Check sheet for the modelled part. Datum: model origin and axes. Units: mm. Face numbers are marked on the shaded views. Round coordinates to 2 decimals unless told otherwise and drop trailing zeros. Write each loop counter-clockwise with the first axis right and the second up, starting at its lowest first coordinate (ties: lowest second). Pieces come first, ordered by that corner, then holes.
Item 1: Go/stop test with flat-tipped pins: pin 1 Ø3 at (x, y) = (-20.22, 50.58) entering from +Z; pin 2 Ø6 at (y, z) = (54, -2) entering from +X; pin 3 Ø17.5 at (x, y) = (10, 58) entering from +Z; pin 4 Ø1 at (y, z) = (59, -2) entering from +X. Record where each tip stops, or that it passes through.
Item 2: Cross-section at D-D on z = -4. Enter the section's corners in (x, y).
Item 3: Cross-section at C-C on y = 64.58. Enter the section's corners in (x, z), plus the area to 3 significant figures.
Item 4: Release check for a two-part mould opening along X. For the marked faces 1, 2 and 3 record: +X half, -X half, draft (parallel to the pull), parting line (faces both ways), or undercut.
Item 5: Material ranges on line 1 (X direction, y = 58.5, z = -2.5); line 2 (X direction, y = 56, z = 3.75); line 3 (X direction, y = 56, z = -3), recorded low to high.
Item 6: Cross-section at B-B on z = 4.25. Enter the section's corners in (x, y).
Item 7: Cross-section at A-A on x = -20.22. Enter the section's corners in (y, z), plus the area to 3 significant figures.
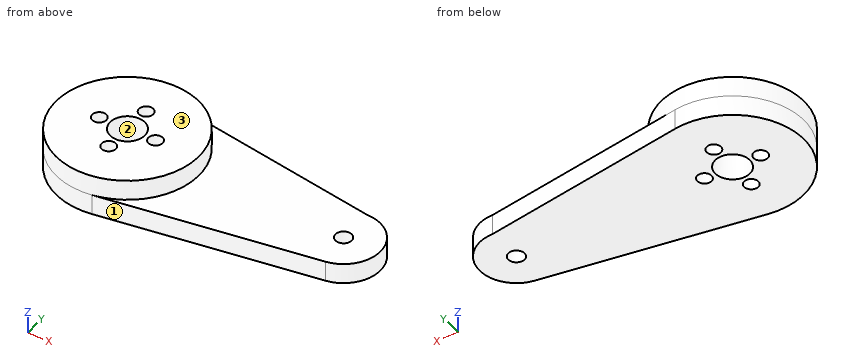
from build123d import *

# Parameters (mm, degrees)
SKETCH2_R           = 4.25
SKETCH2_R_2         = 2
BOSS_EXTRUDE1_DEPTH = 5
SKETCH_1_R          = 1.75
CUT_EXTRUDE_1_DEPTH = 10
EXTRUDE_START       = 5
SKETCH_2_R          = 17.5
SKETCH_2_R_2        = 1.75
SKETCH_2_R_3        = 4.25
EXTRUDE_1_DEPTH     = 5


with BuildPart() as part:
    # Sketch2 → Boss-Extrude1 (new body)
    with BuildSketch(Plane.XY):
        with BuildLine():
            Line((-17.328874887, 74.839530577), (33.78000003, 66.278338859))
            ThreePointArc((33.78000003, 66.278338859), (42.753857637, 57.963816533), (35.14697315, 48.382756557))
            Line((35.14697315, 48.382756557), (-17.561996681, 40.283034413))
            ThreePointArc((-17.561996681, 40.283034413), (-37.719601772, 57.698054173), (-17.328874887, 74.839530577))
        make_face()
        with Locations((-20.21999997, 57.58)):
            Circle(SKETCH2_R, mode=Mode.SUBTRACT)
        with Locations((33.78000003, 57.278338859)):
            Circle(SKETCH2_R_2, mode=Mode.SUBTRACT)
    extrude(amount=-BOSS_EXTRUDE1_DEPTH)

    # 草图1 → 切除-拉伸1 (cut)
    with BuildSketch(Plane.XY):
        with Locations((-13.21999997, 57.58)):
            Circle(SKETCH_1_R)
        with Locations((-27.21999997, 57.58)):
            Circle(SKETCH_1_R)
        with Locations((-20.21999997, 64.58)):
            Circle(SKETCH_1_R)
        with Locations((-20.21999997, 50.58)):
            Circle(SKETCH_1_R)
    extrude(amount=-CUT_EXTRUDE_1_DEPTH, mode=Mode.SUBTRACT)

    # 草图2 → 凸台-拉伸1 (add)
    with BuildSketch(Plane.XY.offset(EXTRUDE_START)):
        with Locations((-20.21999997, 57.58)):
            Circle(SKETCH_2_R)
        with Locations((-27.21999997, 57.58)):
            Circle(SKETCH_2_R_2, mode=Mode.SUBTRACT)
        with Locations((-20.21999997, 50.58)):
            Circle(SKETCH_2_R_2, mode=Mode.SUBTRACT)
        with Locations((-13.21999997, 57.58)):
            Circle(SKETCH_2_R_2, mode=Mode.SUBTRACT)
        with Locations((-20.21999997, 64.58)):
            Circle(SKETCH_2_R_2, mode=Mode.SUBTRACT)
        with Locations((-20.21999997, 57.58)):
            Circle(SKETCH_2_R_3, mode=Mode.SUBTRACT)
    extrude(amount=-EXTRUDE_1_DEPTH)


solid = part.part
Response values:
1. pin 1: passes through
1. pin 2: stops at x = 42.78
1. pin 3: stops at z = 0
1. pin 4: stops at x = 42.7
2. outline: (-17.56, 40.28) - (35.15, 48.38) arc R9 ccw to (33.78, 66.28) - (-17.33, 74.84) arc R17.5 ccw (long way) to start; hole circle Ø3.5 at (-27.22, 57.58); hole circle Ø8.5 at (-20.22, 57.58); hole circle Ø3.5 at (-20.22, 50.58); hole circle Ø3.5 at (-20.22, 64.58); hole circle Ø3.5 at (-13.22, 57.58); hole circle Ø4 at (33.78, 57.28)
3. outline: (-36.26, -5) - (-21.97, -5) - (-21.97, 5) - (-36.26, 5) - close; (-18.47, -5) - (39.04, -5) - (39.04, 0) - (-4.18, 0) - (-4.18, 5) - (-18.47, 5) - close
3. area: 502 mm2
4. face 1: +X half
4. face 2: undercut
4. face 3: draft
5. line 1: x = -37.7 to -28.71, -25.73 to -24.37, -16.07 to -14.71, -11.73 to 32.2, 35.36 to 42.7
5. line 2: x = -37.65 to -27.97, -26.47 to -24.17, -16.27 to -13.97, -12.47 to -2.79
5. line 3: x = -37.65 to -27.97, -26.47 to -24.17, -16.27 to -13.97, -12.47 to 32.24, 35.32 to 42.69
6. outline: circle Ø35 at (-20.22, 57.58); hole circle Ø3.5 at (-27.22, 57.58); hole circle Ø8.5 at (-20.22, 57.58); hole circle Ø3.5 at (-20.22, 50.58); hole circle Ø3.5 at (-20.22, 64.58); hole circle Ø3.5 at (-13.22, 57.58)
7. outline: (40.08, -5) - (48.83, -5) - (48.83, 5) - (40.08, 5) - close; (52.33, -5) - (53.33, -5) - (53.33, 5) - (52.33, 5) - close; (61.83, -5) - (62.83, -5) - (62.83, 5) - (61.83, 5) - close; (66.33, -5) - (75.08, -5) - (75.08, 5) - (66.33, 5) - close
7. area: 195 mm2
